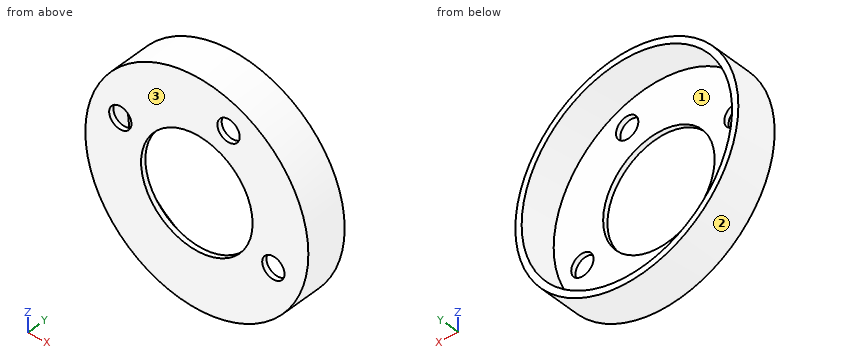
from build123d import *

# Parameters (mm, degrees)
SKETCH1_R           = 35
SKETCH1_R_2         = 17.5
SKETCH1_R_3         = 3.5
BOSS_EXTRUDE1_DEPTH = 12.954
SKETCH2_R           = 33.02
CUT_EXTRUDE1_DEPTH  = 11.43


with BuildPart() as part:
    # Sketch1 → Boss-Extrude1 (new body)
    with BuildSketch(Plane(origin=(0, 0, 0), x_dir=(1, 0, 0), z_dir=(0, 1, 0))):
        Circle(SKETCH1_R)
        Circle(SKETCH1_R_2, mode=Mode.SUBTRACT)
        with Locations((-24.023795501, -9.950801949)):
            Circle(SKETCH1_R_3, mode=Mode.SUBTRACT)
        with Locations((24.018239985, 9.948012748)):
            Circle(SKETCH1_R_3, mode=Mode.SUBTRACT)
        with Locations((9.950974523, -24.02421215)):
            Circle(SKETCH1_R_3, mode=Mode.SUBTRACT)
    extrude(amount=BOSS_EXTRUDE1_DEPTH)

    # Sketch2 → Cut-Extrude1 (cut)
    with BuildSketch(Plane(origin=(0, 12.954, 0), x_dir=(1, 0, 0), z_dir=(0, 1, 0))):
        Circle(SKETCH2_R)
    extrude(amount=-CUT_EXTRUDE1_DEPTH, mode=Mode.SUBTRACT)


solid = part.part
Verification items for the finished model (mm, model axes). Face numbers are marked on the shaded views. Round coordinates to 2 decimals unless told otherwise and drop trailing zeros. Order: outer loops, then holes, each group sorted by start corner. A loop starts at its lowest first (then second) coordinate and runs counter-clockwise, first axis right, second up. Notation, with made-up numbers: (23, 10.5) -> (63, 10.5) arc R27 cw to (63, 49.5) -> close; hole circle Ø5 at (-11.75, 24.5). An arc over 180 degrees is marked (long way). Put each result on its own line as item: value.
1) Section check C-C (z = -9). Record the cut outline in (x, y), then the cut area to 3 significant figures.
Final values:
outline: (-33.82, 0) -> (-15.01, 0) -> (-15.01, 1.52) -> (-31.77, 1.52) -> (-31.77, 12.95) -> (-33.82, 12.95) -> close; (15.01, 0) -> (20.65, 0) -> (20.65, 1.52) -> (15.01, 1.52) -> close; (27.39, 0) -> (33.82, 0) -> (33.82, 12.95) -> (31.77, 12.95) -> (31.77, 1.52) -> (27.39, 1.52) -> close
area: 94.0 mm^2
2) Depth check by flat-ended pin: pin 1 (3 mm diameter, centred on x = -11, z = 12.5, fed in from +Y); pin 2 (4 mm diameter, centred on x = -23, y = 6, fed in from +Z); pin 3 (9 mm diameter, centred on x = 24.02, z = -9.95, fed in from -Y); pin 4 (4 mm diameter, centred on x = -7.5, y = 1.5, fed in from +Z). Enter the tip coordinate at first touch or a pass-through.
Final values:
pin 1: stops at y = 1.52
pin 2: stops at z = 28
pin 3: stops at y = 0
pin 4: stops at z = 34.57
3) Section check B-B (x = 0). Record the cut outline in (y, z).
Final values:
outline: (0, -35) -> (12.95, -35) -> (12.95, -33.02) -> (1.52, -33.02) -> (1.52, -17.5) -> (0, -17.5) -> close; (0, 17.5) -> (1.52, 17.5) -> (1.52, 33.02) -> (12.95, 33.02) -> (12.95, 35) -> (0, 35) -> close
4) Mould release check, pull along X, two halves, no side actions. Record for the marked faces 1, 2 and 3: +X half, -X half, draft (parallel to the pull), parting line (faces both ways), or undercut.
Final values:
face 1: undercut
face 2: parting line
face 3: draft
5) Section check D-D (x = 7.5). Record the cut outline in (y, z), then the cut area to 3 significant figures.
Final values:
outline: (0, -34.19) -> (12.95, -34.19) -> (12.95, -32.16) -> (1.52, -32.16) -> (1.52, -15.81) -> (0, -15.81) -> close; (0, 15.81) -> (1.52, 15.81) -> (1.52, 21.53) -> (0, 21.53) -> close; (0, 26.52) -> (1.52, 26.52) -> (1.52, 32.16) -> (12.95, 32.16) -> (12.95, 34.19) -> (0, 34.19) -> close
area: 94.8 mm^2
6) Section check A-A (z = 0). Record the cut outline in (x, y).
Final values:
outline: (-35, 0) -> (-17.5, 0) -> (-17.5, 1.52) -> (-33.02, 1.52) -> (-33.02, 12.95) -> (-35, 12.95) -> close; (17.5, 0) -> (35, 0) -> (35, 12.95) -> (33.02, 12.95) -> (33.02, 1.52) -> (17.5, 1.52) -> close
7) Material ranges on line 1 (X direction, y = 0.9, z = 0); line 2 (Y direction, x = -20.5, z = 1), recorded low to high.
Final values:
line 1: x = -35 to -17.5, 17.5 to 35
line 2: y = 0 to 1.52
